from build123d import *

# Parameters (mm, degrees)
F1_DEPTH = 12.7


with BuildPart() as f1:
    # F0 (on Front) → F1 (new body)
    with BuildSketch(Plane.XZ):
        with BuildLine():
            Line((-10.867325, 6.717781), (-21.023455, 6.437397))
            Line((-21.023455, 6.437397), (-20.743071, -3.718733))
            Line((-20.743071, -3.718733), (-17.696232, -3.634618))
            ThreePointArc((-17.696232, -3.634618), (-12.216315, -6.0243), (-17.55604, -8.712683))
            Line((-17.55604, -8.712683), (-20.602879, -8.796799))
            Line((-20.602879, -8.796799), (-20.322495, -18.952929))
            Line((-20.322495, -18.952929), (-10.166365, -18.672545))
            Line((-10.166365, -18.672545), (-5.088299, -18.532353))
            Line((-5.088299, -18.532353), (5.067831, -18.251969))
            Line((5.067831, -18.251969), (4.790878, -8.220124))
            Line((4.790878, -8.220124), (4.647255, -3.017773))
            Line((4.647255, -3.017773), (4.366871, 7.138357))
            Line((4.366871, 7.138357), (-5.78926, 6.857973))
            Line((-5.78926, 6.857973), (-5.705144, 3.811134))
            ThreePointArc((-5.705144, 3.811134), (-8.094826, -1.668783), (-10.78321, 3.670942))
            Line((-10.78321, 3.670942), (-10.867325, 6.717781))
        make_face()
        with BuildLine():
            Line((-5.088299, -18.532353), (-10.166365, -18.672545))
            Line((-10.166365, -18.672545), (-10.082249, -21.719384))
            ThreePointArc((-10.082249, -21.719384), (-7.393866, -27.059109), (-5.004184, -21.579192))
            Line((-5.004184, -21.579192), (-5.088299, -18.532353))
        make_face()
        with BuildLine():
            Line((7.694094, -2.933658), (4.647255, -3.017773))
            Line((4.647255, -3.017773), (4.790878, -8.220124))
            Line((4.790878, -8.220124), (7.837717, -8.136009))
            ThreePointArc((7.837717, -8.136009), (13.098589, -5.387612), (7.694094, -2.933658))
        make_face()
    extrude(amount=F1_DEPTH)


solid = f1.part
Here's how the part is built. I have some questions about the finished solid (model axes, mm). Coordinates: 2 decimals unless noted, no trailing zeros. Write each loop counter-clockwise with the first axis right and the second up, starting at its lowest first coordinate (ties: lowest second). Pieces come first, ordered by that corner, then holes. Notation, with made-up numbers: (-8, -31) - (34, -31) arc R9 cw to (34, -19) - close; hole circle Ø11 at (10, 47.25). An arc over 180 degrees is marked (long way). Use one line per item in the form item = value.
1) Suppose I cut it at D-D, the plane x = 6. Write out the boundary of the cut face in (y, z).
Solved:
outline = (-12.7, -8.19) - (0, -8.19) - (0, -2.98) - (-12.7, -2.98) - close
2) Suppose I cut it at B-B, the plane y = -0.75. Write out the boundary of the cut face in (x, z) (1 decimal), plus the area to 3 significant figures.
Solved:
outline = (-21, 6.4) - (-20.7, -3.7) - (-17.7, -3.6) arc R3.3 cw (long way) to (-17.6, -8.7) - (-20.6, -8.8) - (-20.3, -19) - (-10.2, -18.7) - (-10.1, -21.7) arc R3.3 ccw (long way) to (-5, -21.6) - (-5.1, -18.5) - (5.1, -18.3) - (4.8, -8.2) - (7.8, -8.1) arc R3.3 ccw (long way) to (7.7, -2.9) - (4.6, -3) - (4.4, 7.1) - (-5.8, 6.9) - (-5.7, 3.8) arc R3.3 cw (long way) to (-10.8, 3.7) - (-10.9, 6.7) - close
area = 645 mm2
3) I need wall thicknesses on line 1 (Z direction, x = 10, y = -2.75); line 2 (X direction, y = -1, z = 5); line 3 (X direction, y = -6.5, z = -9). Which ranges of each line are inside material? Lowest first, please.
Solved:
line_1 = -8.77 to -2.18
line_2 = -20.98 to -10.82, -5.74 to 4.43
line_3 = -20.6 to -17.12, -13.91 to 4.81
4) Suppose I cut it at A-A, the plane z = -0.5. Write out the boundary of the cut face in (x, y), plus the area to 3 significant figures.
Solved:
outline = (-20.83, -12.7) - (-10.71, -12.7) - (-10.71, 0) - (-20.83, 0) - close; (-5.66, -12.7) - (4.58, -12.7) - (4.58, 0) - (-5.66, 0) - close
area = 259 mm2
5) I'm going to push flat-ended pins straight in: P1, Ø6, axis at y = -9.5, z = -3.5, coming from the -X side; P2, Ø5, axis at y = -8.5, z = 3.5, coming from the +X side; P3, Ø5, axis at y = -7, z = -17, coming from the +X side. Where does each tip first touch, or does it pass through?
Solved:
P1 = -20.83
P2 = 4.54
P3 = 5.07
6) Thinking about a two-plate mould opening in Z: for faces 1 (the cylindrical face through (13.1, -6.3, -5.5)), 2 (the cylindrical face through (-12.22, -6.26, -5.92)), which applies, released by +Z, released by -Z, zero draft, split by the parting line, or undercut?
Solved:
face_1 = split by the parting line
face_2 = undercut
7) Suppose I cut it at C-C, the plane x = -19. Write out the boundary of the cut face in (y, z).
Solved:
outline = (-12.7, -18.92) - (0, -18.92) - (0, -8.75) - (-12.7, -8.75) - close; (-12.7, -3.67) - (0, -3.67) - (0, 6.49) - (-12.7, 6.49) - close
